```python
from build123d import *

# Parameters (mm, degrees)
SKETCH_W            = 54
SKETCH_H            = 44
PAD_DEPTH           = 82.5
SKETCH001_W         = 32
SKETCH001_H         = 44
POCKET_DEPTH        = 76.5
SKETCH002_R         = 1.6
HOLE_DEPTH          = 50
HOLE001_DEPTH       = 25
HOLE001_TIPS_R      = 1.6
SKETCH003_R         = 1
HOLE002_DEPTH       = 12
HOLE003_D           = 3.5
HOLE003_DEPTH       = 25
HOLE003_CBORE_D     = 6
HOLE003_CBORE_DEPTH = 6
HOLE003_TIPS_R      = 1.75
CHAMFER_SIZE        = 2


with BuildPart() as part:
    # Sketch → Pad (new body)
    with BuildSketch(Plane.XY):
        Rectangle(SKETCH_W, SKETCH_H)
    extrude(amount=PAD_DEPTH)

    # Sketch001 (on Face6 of Pad) → Pocket (cut)
    with BuildSketch(Plane.XY.offset(82.5)):
        with Locations((0, 11)):
            Rectangle(SKETCH001_W, SKETCH001_H)
    extrude(amount=-POCKET_DEPTH, mode=Mode.SUBTRACT)

    # Sketch002 → Hole (cut)
    with BuildSketch(Plane.YZ):
        with Locations((0, 41)):
            Circle(SKETCH002_R)
        with Locations((13.75, 41)):
            Circle(SKETCH002_R)
        with Locations((0, 54.75)):
            Circle(SKETCH002_R)
        with Locations((0, 27.25)):
            Circle(SKETCH002_R)
        with Locations((-13.75, 41)):
            Circle(SKETCH002_R)
    extrude(amount=-HOLE_DEPTH, mode=Mode.SUBTRACT)

    # Sketch002 → Hole001 (cut)
    with BuildSketch(Plane.YZ):
        with Locations((0, 41)):
            Circle(SKETCH002_R)
        with Locations((13.75, 41)):
            Circle(SKETCH002_R)
        with Locations((0, 54.75)):
            Circle(SKETCH002_R)
        with Locations((0, 27.25)):
            Circle(SKETCH002_R)
        with Locations((-13.75, 41)):
            Circle(SKETCH002_R)
    extrude(amount=HOLE001_DEPTH, mode=Mode.SUBTRACT)

    # Hole001 tips → Hole001 tip 1 section 0
    with BuildSketch(Plane.YZ.offset(25), mode=Mode.PRIVATE) as hole001_tip_1_s0:
        with Locations((0, 41)):
            Circle(HOLE001_TIPS_R)
    loft([hole001_tip_1_s0.sketch, Vertex(25.961377, 0, 41)], mode=Mode.SUBTRACT)

    # Hole001 tips → Hole001 tip 2 section 0
    with BuildSketch(Plane.YZ.offset(25), mode=Mode.PRIVATE) as hole001_tip_2_s0:
        with Locations((13.75, 41)):
            Circle(HOLE001_TIPS_R)
    loft([hole001_tip_2_s0.sketch, Vertex(25.961377, 13.75, 41)], mode=Mode.SUBTRACT)

    # Hole001 tips → Hole001 tip 3 section 0
    with BuildSketch(Plane.YZ.offset(25), mode=Mode.PRIVATE) as hole001_tip_3_s0:
        with Locations((0, 54.75)):
            Circle(HOLE001_TIPS_R)
    loft([hole001_tip_3_s0.sketch, Vertex(25.961377, 0, 54.75)], mode=Mode.SUBTRACT)

    # Hole001 tips → Hole001 tip 4 section 0
    with BuildSketch(Plane.YZ.offset(25), mode=Mode.PRIVATE) as hole001_tip_4_s0:
        with Locations((0, 27.25)):
            Circle(HOLE001_TIPS_R)
    loft([hole001_tip_4_s0.sketch, Vertex(25.961377, 0, 27.25)], mode=Mode.SUBTRACT)

    # Hole001 tips → Hole001 tip 5 section 0
    with BuildSketch(Plane.YZ.offset(25), mode=Mode.PRIVATE) as hole001_tip_5_s0:
        with Locations((-13.75, 41)):
            Circle(HOLE001_TIPS_R)
    loft([hole001_tip_5_s0.sketch, Vertex(25.961377, -13.75, 41)], mode=Mode.SUBTRACT)

    # Sketch003 → Hole002 (cut)
    with BuildSketch(Plane.XY):
        with Locations((-13, 18.5)):
            Circle(SKETCH003_R)
        with Locations((13, 18.5)):
            Circle(SKETCH003_R)
        with Locations((13, -18.5)):
            Circle(SKETCH003_R)
        with Locations((-13, -18.5)):
            Circle(SKETCH003_R)
    extrude(amount=-HOLE002_DEPTH, mode=Mode.SUBTRACT)

    # Hole003
    with Locations(Plane.XZ.offset(22)):
        with Locations((0, 56), (10, 79.7), (-10, 79.7)):
            CounterBoreHole(HOLE003_D / 2, HOLE003_CBORE_D / 2, HOLE003_CBORE_DEPTH, depth=HOLE003_DEPTH)

    # Hole003 tips → Hole003 tip 1 section 0
    with BuildSketch(Plane.XZ.offset(-3), mode=Mode.PRIVATE) as hole003_tip_1_s0:
        with Locations((0, 56)):
            Circle(HOLE003_TIPS_R)
    loft([hole003_tip_1_s0.sketch, Vertex(0, 4.051506, 56)], mode=Mode.SUBTRACT)

    # Hole003 tips → Hole003 tip 2 section 0
    with BuildSketch(Plane.XZ.offset(-3), mode=Mode.PRIVATE) as hole003_tip_2_s0:
        with Locations((10, 79.7)):
            Circle(HOLE003_TIPS_R)
    loft([hole003_tip_2_s0.sketch, Vertex(10, 4.051506, 79.7)], mode=Mode.SUBTRACT)

    # Hole003 tips → Hole003 tip 3 section 0
    with BuildSketch(Plane.XZ.offset(-3), mode=Mode.PRIVATE) as hole003_tip_3_s0:
        with Locations((-10, 79.7)):
            Circle(HOLE003_TIPS_R)
    loft([hole003_tip_3_s0.sketch, Vertex(-10, 4.051506, 79.7)], mode=Mode.SUBTRACT)

    # Chamfer
    chamfer_edges = [part.edges().sort_by_distance(p)[0] for p in [
        (-27, 0, 0),
        (0, 22, 0),
        (27, 0, 0),
        (0, -22, 0),
    ]]
    chamfer(chamfer_edges, length=CHAMFER_SIZE)


solid = part.part
```
Here's how the part is built. I have some questions about the finished solid (model axes, mm). A direction names the side the tool comes from. Give positions to 0.01 mm unless a question says otherwise; leave off trailing zeros. Order: outer loops, then holes, each group sorted by start corner. A loop starts at its lowest first (then second) coordinate and runs counter-clockwise, first axis right, second up. Notation, with made-up numbers: (-29.5, 57.5) - (-14.5, 57.5) arc R25 ccw to (-14.5, 88.5) - close; hole circle Ø8 at (84, 65.25). An arc over 180 degrees is marked (long way). Answer as a JSON object with one key per item and string values. Group by question number.
Item 1: For P1, Ø2, axis at x = 10, z = 79.7, coming from the +Y side; P2, Ø12, axis at x = 11.5, z = 70, coming from the +Y side; P3, Ø3, axis at x = -2, z = 38, coming from the +Y side; P4, Ø1.9, axis at y = 13.75, z = 41, coming from the -X side, each with a flat end and sliding along its axis, tell me the tip position at first contact or that it passes through.
Item 2: If we section it at B-B on z = 46: Please give me the cut outline in (x, y), and give its area (3 significant figures).
Item 3: Which directions (+Z, -Z, +X, -X, +Y, -Y) give clear straight access to the entire face, cutting with the end or side of a thin tool? Please do faces 1 (the flat face through (2, -16, 56)), 2 (the cylindrical face through (20.4, 12.5, 40)), 3 (the flat face through (0, 6, 6)).
Item 4: If we section it at A-A on x = 10: Please give me the cut outline in (y, z), and give its area (3 significant figures).
Item 5: Please list where these lines run through material, in increasing order: probe 1 along Z at (x, y) = (-19, 0); probe 2 along X at (y, z) = (-13.3, 79.7); probe 3 along Z at (x, y) = (-22, -0.5).
Item 6: If we section it at C-C on y = 9: Please give me the cut outline in (x, z), and give its area (3 significant figures).
Item 7: If we mould it in two halves opening along X, with no side actions, what happens to faces 4 (the flat face through (-16, 5, 45)), 5 (the flat face through (0, -21, 1)), 6 (the flat face through (27, 0, 42))? For each: pulls with the +X half, pulls with the -X half, needs draft (parallel to the pull), parting line crosses it, or undercut.
Result set:
{
 "1": {"P1": "through", "P2": "y = 22", "P3": "y = -11", "P4": "x = 25.39"},
 "2": {"outline": "(-27, -22) - (27, -22) - (27, 22) - (16, 22) - (16, -11) - (-16, -11) - (-16, 22) - (-27, 22) - close", "area": "1,320 mm²"},
 "3": {"face 1": "-Y", "face 2": "-X", "face 3": "+Z, +Y"},
 "4": {"outline": "(-22, 2) - (-20, 0) - (20, 0) - (22, 2) - (22, 6) - (-11, 6) - (-11, 77.95) - (-16, 77.95) - (-16, 76.7) - (-22, 76.7) - close; (-16, 81.45) - (-11, 81.45) - (-11, 82.5) - (-16, 82.5) - close; hole circle Ø3.2 at (-13.75, 41)", "area": "1,040 mm²"},
 "5": {"probe 1": "0 to 25.65, 28.85 to 39.4, 42.6 to 53.15, 56.35 to 82.5", "probe 2": "-27 to -11.75, -8.25 to 8.25, 11.75 to 27", "probe 3": "0 to 25.73, 28.77 to 39.48, 42.52 to 53.23, 56.27 to 82.5"},
 "6": {"outline": "(-27, 2) - (-25, 0) - (25, 0) - (27, 2) - (27, 82.5) - (16, 82.5) - (16, 6) - (-16, 6) - (-16, 82.5) - (-27, 82.5) - close", "area": "2,000 mm²"},
 "7": {"face 4": "undercut", "face 5": "needs draft", "face 6": "pulls with the +X half"}
}
